Autodesk Inventor part; units mm, degrees
ref_plane "YZ Plane" through (0, 0, 0) normal (1, 0, 0) x (0, 1, 0)
ref_plane "XZ Plane" through (0, 0, 0) normal (0, 1, 0) x (-1, 0, 0)
ref_plane "XY Plane" through (0, 0, 0) normal (0, 0, 1) x (1, 0, 0)
sketch "Sketch2" plane through (0, 0, 0) normal (0, 1, 0) x (-1, 0, 0)
  line L0 (9.271, 3.81) -> (-9.271, 3.81)
  line L1 (-9.271, 3.81) -> (-9.271, -3.81)
  line L2 (-9.271, -3.81) -> (9.271, -3.81)
  line L3 (9.271, -3.81) -> (9.271, 3.81)
  line L4 (9.271, 3.81) -> (-9.271, -3.81) construction
  line L5 (-9.271, 3.81) -> (9.271, -3.81) construction
  point P0 (0, 0)
  dimension "d3" = 18.542
  dimension "d4" = 7.62
extrude "Extrusion2" add sketch "Sketch2" along normal blind 114.3
sketch "Sketch3" plane through (0, 114.3, 0) normal (0, 1, 0) x (1, 0, 0)
  point P0 (0, 0)
sketch "Sketch4" plane through (0, 0, 0) normal (0, -1, 0) x (1, 0, 0)
  line L0 (-10.541, -5.08) -> (10.541, -5.08)
  line L1 (10.541, -5.08) -> (10.541, 5.08)
  line L2 (10.541, 5.08) -> (-10.541, 5.08)
  line L3 (-10.541, 5.08) -> (-10.541, -5.08)
  line L4 (-10.541, -5.08) -> (10.541, 5.08) construction
  line L5 (10.541, -5.08) -> (-10.541, 5.08) construction
  point P0 (0, 0)
  dimension "d7" = 21.082
  dimension "d8" = 10.16
extrude "Extrusion3" add sketch "Sketch4" against normal blind 93.1926
hole "Hole1" at (0, 114.3, 0) direction (0, -1, 0) diameter 3.302 end through all
sketch "Sketch5" plane through (0, 114.3, 0) normal (0, 1, 0) x (1, 0, 0)
  line L0 (7.62, -2.54) -> (-7.62, -2.54)
  line L1 (-7.62, -2.54) -> (-7.62, 2.54)
  line L2 (-7.62, 2.54) -> (7.62, 2.54)
  line L3 (7.62, 2.54) -> (7.62, -2.54)
  line L4 (7.62, -2.54) -> (-7.62, 2.54) construction
  line L5 (-7.62, -2.54) -> (7.62, 2.54) construction
  point P0 (0, 0)
  dimension "d18" = 15.24
  dimension "d19" = 5.08
extrude "Extrusion4" cut sketch "Sketch5" against normal blind 105.8926
sketch "Sketch6" plane through (0, 114.3, 0) normal (0, 1, 0) x (1, 0, 0)
  line L0 (14.2875, -6.35) -> (-14.2875, -6.35)
  line L1 (-14.2875, -6.35) -> (-14.2875, 6.35)
  line L2 (-14.2875, 6.35) -> (14.2875, 6.35)
  line L3 (14.2875, 6.35) -> (14.2875, -6.35)
  line L4 (14.2875, -6.35) -> (-14.2875, 6.35) construction
  line L5 (-14.2875, -6.35) -> (14.2875, 6.35) construction
  point P0 (0, 0)
extrude "Extrusion5" cut sketch "Sketch6" against normal blind 11.1125
sketch "Sketch7" plane through (-10.541, 0, 5.08) normal (0, 0, 1) x (1, 0, 0)
  line L0 (3.6195, 82.55) -> (17.4625, 82.55)
  line L1 (17.4625, 82.55) -> (17.4625, 57.15)
  line L2 (17.4625, 57.15) -> (3.6195, 57.15)
  line L3 (3.6195, 57.15) -> (3.6195, 82.55)
  line L4 (3.6195, 82.55) -> (17.4625, 57.15) construction
  line L5 (17.4625, 82.55) -> (3.6195, 57.15) construction
  line L6 (3.6195, 15.875) -> (17.4625, 15.875)
  line L7 (17.4625, 15.875) -> (17.4625, 41.275)
  line L8 (17.4625, 41.275) -> (3.6195, 41.275)
  line L9 (3.6195, 41.275) -> (3.6195, 15.875)
  line L10 (3.6195, 15.875) -> (17.4625, 41.275) construction
  line L11 (17.4625, 15.875) -> (3.6195, 41.275) construction
  point P0 (10.541, 0)
  point P1 (10.541, 69.85)
  point P2 (10.541, 28.575)
extrude "Extrusion6" cut sketch "Sketch7" against normal blind 25.4
properties part number "Pizza2"
Could you check a few things on this model? Use its own coordinates, in mm. A direction names the side the tool comes from. Give positions to 0.01 mm unless a question says otherwise; leave off trailing zeros. Loops run counter-clockwise (first coordinate to the right, second up) from the corner with the lowest first, then second, coordinate; pieces in that order, holes last. Notation, with made-up numbers: (61.5, 72.25) - (96.5, 72.25) arc R15 ccw to (96.5, 86.25) - close; hole circle Ø3 at (7, 26). An arc over 180 degrees is marked (long way). Use one line per item in the form item = value.
1. I'm going to push flat-ended pins straight in: pin 1 Ø8 at (x, y) = (0, 96) entering from +Z; pin 2 Ø4.5 at (x, y) = (2, 61) entering from -Z; pin 3 Ø5 at (x, y) = (2, 98.5) entering from -Z. Where does each tip first touch, or does it pass through?
Response values:
pin_1 = 5.08
pin_2 = through
pin_3 = -3.81
2. Thinking about a two-plate mould opening in X: for faces 1 (the face through (0, 82.55, 4)), 2 (the face through (0, 98, 3.81)), 3 (the face through (10.541, 46, 0)), which applies, released by +X, released by -X, zero draft, split by the parting line, or undercut?
Response values:
face_1 = undercut
face_2 = zero draft
face_3 = released by +X
3. On a 3-axis mill with a long thin cutter (end or side, diameter ignored), from which of +Z, -Z, +X, -X, +Y, -Y can I reach the whole of each face in a straight line? I mean faces 4 (the face through (0, 0, -2)), 5 (the face through (0, 56, -2.54)), 6 (the face through (0, 46, 5.08)), 7 (the face through (0, 98, -3.81)), 8 (the face through (-6.922, 29, -4)). Say none if no direction works.
Response values:
face_4 = +Z, -Z, +X, -X, -Y
face_5 = +Y
face_6 = +Z, +X, -X, +Y, -Y
face_7 = -Z, +X, -X, +Y
face_8 = +Z, -Z
4. I want a section at C-C (y = 39). Please give me the cut outline in (x, z).
Response values:
outline = (-10.54, -5.08) - (-6.92, -5.08) - (-6.92, -2.54) - (-7.62, -2.54) - (-7.62, 2.54) - (-6.92, 2.54) - (-6.92, 5.08) - (-10.54, 5.08) - close; (6.92, -5.08) - (10.54, -5.08) - (10.54, 5.08) - (6.92, 5.08) - (6.92, 2.54) - (7.62, 2.54) - (7.62, -2.54) - (6.92, -2.54) - close
5. I want a section at B-B (x = -5.25). Give the number of separate pieces and of enclosed holes in the cut face, and give its area (3 significant figures).
Response values:
separate_pieces = 5
enclosed_holes = 0
area = 283 mm²
6. I want a section at A-A (z = 0). Please give me the cut outline in (x, y).
Response values:
outline = (-10.54, 0) - (-1.65, 0) - (-1.65, 8.41) - (-7.62, 8.41) - (-7.62, 103.19) - (-9.27, 103.19) - (-9.27, 93.19) - (-10.54, 93.19) - close; (1.65, 0) - (10.54, 0) - (10.54, 93.19) - (9.27, 93.19) - (9.27, 103.19) - (7.62, 103.19) - (7.62, 8.41) - (1.65, 8.41) - close
7. I need wall thicknesses on probe 1 along Y at (x, z) = (-1.5, 4.5) (3 decimals); probe 2 along Z at (x, y) = (-6, 55); probe 3 along X at (y, z) = (2, 0). Which ranges of each line are inside material? Lowest first, please.
Response values:
probe_1 = 0 to 15.875, 41.275 to 57.15, 82.55 to 93.193
probe_2 = -5.08 to -2.54, 2.54 to 5.08
probe_3 = -10.54 to -1.65, 1.65 to 10.54
